```python
from build123d import *

# Parameters (mm, degrees)
BOSS_EXTRUDE1_DEPTH = 3
BOSS_EXTRUDE2_DEPTH = 10
SKETCH3_W           = 60
SKETCH3_H           = 43
CUT_EXTRUDE1_DEPTH  = 5
SKETCH4_R           = 2.5
BOSS_EXTRUDE3_DEPTH = 3.5
SKETCH5_R           = 1.3
CUT_EXTRUDE2_DEPTH  = 4.5
SKETCH6_R           = 1.3
CUT_EXTRUDE3_DEPTH  = 4.5
SKETCH7_R           = 1.3
CUT_EXTRUDE4_DEPTH  = 4.5
SKETCH8_R           = 1.3
CUT_EXTRUDE5_DEPTH  = 4.5
SKETCH9_R           = 3.1
CUT_EXTRUDE6_DEPTH  = 4.5
SKETCH10_R          = 2.5
SKETCH10_R_2        = 1.15
BOSS_EXTRUDE4_DEPTH = 8
SKETCH12_W          = 7
SKETCH12_H          = 7
BOSS_EXTRUDE5_DEPTH = 10
FILLET1_R           = 3
SKETCH13_R          = 1.3
CUT_EXTRUDE7_DEPTH  = 9


with BuildPart() as part:
    # Sketch1 → Boss-Extrude1 (new body)
    with BuildSketch(Plane(origin=(0, 0, 0), x_dir=(1, 0, 0), z_dir=(0, 1, 0))):
        with BuildLine():
            Line((70, 10), (70, -10))
            ThreePointArc((70, -10), (64.142135624, -24.142135624), (50, -30))
            Line((50, -30), (-50, -30))
            ThreePointArc((-50, -30), (-64.142135624, -24.142135624), (-70, -10))
            Line((-70, -10), (-70, 10))
            ThreePointArc((-70, 10), (-64.142135624, 24.142135624), (-50, 30))
            Line((-50, 30), (50, 30))
            ThreePointArc((50, 30), (64.142135624, 24.142135624), (70, 10))
        make_face()
    extrude(amount=BOSS_EXTRUDE1_DEPTH)

    # Sketch2 → Boss-Extrude2 (add)
    with BuildSketch(Plane(origin=(0, 3, 0), x_dir=(1, 0, 0), z_dir=(0, 1, 0))):
        with BuildLine():
            Line((-50, 30), (50, 30))
            ThreePointArc((50, 30), (64.142135624, 24.142135624), (70, 10))
            Line((70, 10), (70, -10))
            ThreePointArc((70, -10), (64.142135624, -24.142135624), (50, -30))
            Line((50, -30), (-50, -30))
            ThreePointArc((-50, -30), (-64.142135624, -24.142135624), (-70, -10))
            Line((-70, -10), (-70, 10))
            ThreePointArc((-70, 10), (-64.142135624, 24.142135624), (-50, 30))
        make_face()
        with BuildLine():
            Line((-47, 27), (47, 27))
            ThreePointArc((47, 27), (60.435028843, 21.435028843), (66, 8))
            Line((66, 8), (66, -12))
            ThreePointArc((66, -12), (59.103718437, -22.798043353), (47, -27))
            Line((47, -27), (-47, -27))
            ThreePointArc((-47, -27), (-59.103718437, -22.798043353), (-66, -12))
            Line((-66, -12), (-66, 8))
            ThreePointArc((-66, 8), (-60.435028843, 21.435028843), (-47, 27))
        make_face(mode=Mode.SUBTRACT)
    extrude(amount=BOSS_EXTRUDE2_DEPTH)

    # Sketch3 → Cut-Extrude1 (cut)
    with BuildSketch(Plane(origin=(0, 3, 0), x_dir=(1, 0, 0), z_dir=(0, 1, 0))):
        Rectangle(SKETCH3_W, SKETCH3_H)
    extrude(amount=-CUT_EXTRUDE1_DEPTH, mode=Mode.SUBTRACT)

    # Sketch4 → Boss-Extrude3 (add)
    with BuildSketch(Plane(origin=(0, 3, 0), x_dir=(1, 0, 0), z_dir=(0, 1, 0))):
        with Locations((-33.75, 18.25)):
            Circle(SKETCH4_R)
        with Locations((-33.75, -18.25)):
            Circle(SKETCH4_R)
        with Locations((32.75, -18.25)):
            Circle(SKETCH4_R)
        with Locations((32.75, 18.25)):
            Circle(SKETCH4_R)
    extrude(amount=BOSS_EXTRUDE3_DEPTH)

    # Sketch5 → Cut-Extrude2 (cut)
    with BuildSketch(Plane(origin=(0, 6.5, 0), x_dir=(1, 0, 0), z_dir=(0, 1, 0))):
        with Locations((-33.75, -18.25)):
            Circle(SKETCH5_R)
    extrude(amount=-CUT_EXTRUDE2_DEPTH, mode=Mode.SUBTRACT)

    # Sketch6 → Cut-Extrude3 (cut)
    with BuildSketch(Plane(origin=(0, 6.5, 0), x_dir=(1, 0, 0), z_dir=(0, 1, 0))):
        with Locations((-33.75, 18.25)):
            Circle(SKETCH6_R)
    extrude(amount=-CUT_EXTRUDE3_DEPTH, mode=Mode.SUBTRACT)

    # Sketch7 → Cut-Extrude4 (cut)
    with BuildSketch(Plane(origin=(0, 6.5, 0), x_dir=(1, 0, 0), z_dir=(0, 1, 0))):
        with Locations((32.75, 18.25)):
            Circle(SKETCH7_R)
    extrude(amount=-CUT_EXTRUDE4_DEPTH, mode=Mode.SUBTRACT)

    # Sketch8 → Cut-Extrude5 (cut)
    with BuildSketch(Plane(origin=(0, 6.5, 0), x_dir=(1, 0, 0), z_dir=(0, 1, 0))):
        with Locations((32.75, -18.25)):
            Circle(SKETCH8_R)
    extrude(amount=-CUT_EXTRUDE5_DEPTH, mode=Mode.SUBTRACT)

    # Sketch9 → Cut-Extrude6 (cut)
    with BuildSketch(Plane(origin=(0, 3, 0), x_dir=(1, 0, 0), z_dir=(0, 1, 0))):
        with Locations((-44, 0.1)):
            Circle(SKETCH9_R)
        with Locations((-52.1, 8.2)):
            Circle(SKETCH9_R)
        with Locations((-60.2, 0.1)):
            Circle(SKETCH9_R)
        with Locations((-52.1, -8)):
            Circle(SKETCH9_R)
        Polygon((62.3, 3.2), (54.2, 3.2), (54.2, 5.1), (54.2, 11.3), (48, 11.3), (48, 5.1), (48, 3.2), (46.1, 3.2), (39.9, 3.2), (39.9, -3), (46.1, -3), (48, -3), (48, -4.9), (48, -11.1), (54.2, -11.1), (54.2, -4.9), (54.2, -3), (62.3, -3), align=None)
    extrude(amount=-CUT_EXTRUDE6_DEPTH, mode=Mode.SUBTRACT)

    # Sketch10 → Boss-Extrude4 (add)
    with BuildSketch(Plane(origin=(0, 3, 0), x_dir=(1, 0, 0), z_dir=(0, 1, 0))):
        with Locations((-52.1, -16.1)):
            Circle(SKETCH10_R)
        with Locations((-52.1, -16.1)):
            Circle(SKETCH10_R_2, mode=Mode.SUBTRACT)
        with Locations((-52.1, 16.3)):
            Circle(SKETCH10_R)
        with Locations((-52.1, 16.3)):
            Circle(SKETCH10_R_2, mode=Mode.SUBTRACT)
        with Locations((51.1, 16.3)):
            Circle(SKETCH10_R)
        with Locations((51.1, 16.3)):
            Circle(SKETCH10_R_2, mode=Mode.SUBTRACT)
        with Locations((51.1, -16.1)):
            Circle(SKETCH10_R)
        with Locations((51.1, -16.1)):
            Circle(SKETCH10_R_2, mode=Mode.SUBTRACT)
    extrude(amount=BOSS_EXTRUDE4_DEPTH)

    # Sketch12 → Boss-Extrude5 (add)
    with BuildSketch(Plane(origin=(0, 3, 0), x_dir=(1, 0, 0), z_dir=(0, 1, 0))):
        with Locations((-43.5, 23.5)):
            Rectangle(SKETCH12_W, SKETCH12_H)
        with Locations((-43.5, -23.5)):
            Rectangle(SKETCH12_W, SKETCH12_H)
        with Locations((43.5, -23.5)):
            Rectangle(SKETCH12_W, SKETCH12_H)
        with Locations((43.5, 23.5)):
            Rectangle(SKETCH12_W, SKETCH12_H)
    extrude(amount=BOSS_EXTRUDE5_DEPTH)

    # Fillet1
    fillet1_edges = [part.edges().sort_by_distance(p)[0] for p in [
        (70, 0, 0),
        (64.142135624, 0, 24.142135624),
        (0, 0, 30),
        (-64.142135624, 0, 24.142135624),
        (-70, 0, 0),
        (-64.142135624, 0, -24.142135624),
        (0, 0, -30),
        (64.142135624, 0, -24.142135624),
    ]]
    fillet(fillet1_edges, radius=FILLET1_R)

    # Sketch13 → Cut-Extrude7 (cut)
    with BuildSketch(Plane(origin=(0, 13, 0), x_dir=(1, 0, 0), z_dir=(0, 1, 0))):
        with Locations((-43.5, 23.5)):
            Circle(SKETCH13_R)
        with Locations((-43.5, -23.5)):
            Circle(SKETCH13_R)
        with Locations((43.5, -23.5)):
            Circle(SKETCH13_R)
        with Locations((43.5, 23.5)):
            Circle(SKETCH13_R)
    extrude(amount=-CUT_EXTRUDE7_DEPTH, mode=Mode.SUBTRACT)


solid = part.part
```
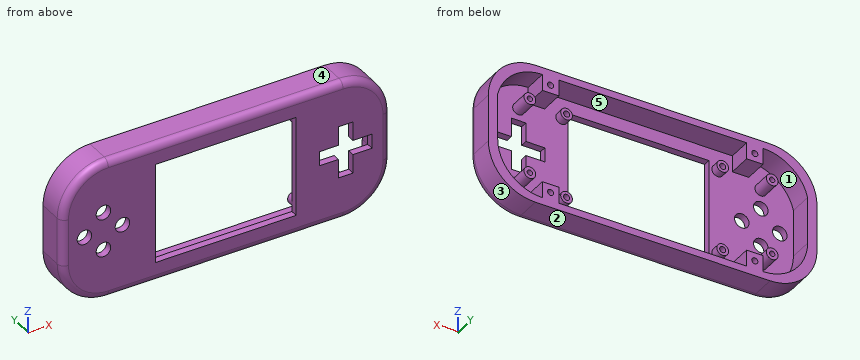
Part model, mm, in its own coordinate system. Face numbers are marked on the shaded views. A direction names the side the tool comes from. Coordinates: 2 decimals unless noted, no trailing zeros. Loops run counter-clockwise (first coordinate to the right, second up) from the corner with the lowest first, then second, coordinate; pieces in that order, holes last. Notation, with made-up numbers: (-35.5, -22.5) - (-29.5, -22.5) arc R21 ccw to (-29.5, -2.5) - close; hole circle Ø5 at (-20.75, -24.5). An arc over 180 degrees is marked (long way). Write item = value, one per line. Start each with the question number.
Item 1: Wall check: L1, parallel to Z at x = -33.75, y = 5.05; L2, parallel to Z at x = 43.5, y = 7.5; L3, parallel to X at y = 10.5, z = 4.5. Give the ranges that are in metal, low to high. Write a range as from..to.
Item 2: Cut at D-D, the plane x = -43.5. Give the cut face in (y, z).
Item 3: Mould opens along X. For the marked faces 1, 2 and 3 say: released by +X, released by -X, zero draft, split by the parting line, or undercut.
Item 4: Cut at B-B, the plane z = 8. Give the cut face in (x, y).
Item 5: Cut at C-C, the plane x = 32.75. Give the cut face in (y, z), and give its area (3 significant figures).
Item 6: Cut at A-A, the plane x = -9.5. Give the cut face in (y, z), and give its area (3 significant figures).
Item 7: Flat gauge pins, fed straight in: pin 1 Ø2 at (y, z) = (8, 23) entering from -X; pin 2 Ø1 at (x, z) = (-47, 0) entering from -Y; pin 3 Ø1.5 at (x, z) = (50.5, -15.5) entering from +Y; pin 4 Ø0.9 at (y, z) = (1, -7.5) entering from +X. Where does each tip first touch, or does it go through?
Item 8: 3-axis set-ups, long thin cutter, end or side, ignore diameter. For the marked faces 4 and 5: which of +Z, -Z, +X, -X, +Y, -Y reach the whole face in a straight line?
The answers:
q1.L1 = -30..-27, -20.75..-19.55, -16.95..-15.75, 15.75..16.95, 19.55..20.75, 27..30
q1.L2 = -30..-24.8, -22.2..-20, 20..22.2, 24.8..30
q1.L3 = -70..-66, 66..70
q2.outline = (0, -27) arc R3 ccw to (3, -30) - (13, -30) - (13, -24.8) - (4, -24.8) - (4, -22.2) - (13, -22.2) - (13, -20) - (3, -20) - (3, -3.16) - (0, -3.16) - close; (0, 2.96) - (3, 2.96) - (3, 20) - (13, 20) - (13, 22.2) - (4, 22.2) - (4, 24.8) - (13, 24.8) - (13, 30) - (3, 30) arc R3 ccw to (0, 27) - close
q3.face_1 = undercut
q3.face_2 = zero draft
q3.face_3 = released by +X
q4.outline = (-70, 3) arc R3 ccw to (-67, 0) - (-55.2, 0) - (-55.2, 3) - (-66, 3) - (-66, 13) - (-70, 13) - close; (-49, 0) - (-30, 0) - (-30, 3) - (-49, 3) - close; (30, 0) - (48, 0) - (48, 3) - (30, 3) - close; (54.2, 0) - (67, 0) arc R3 ccw to (70, 3) - (70, 13) - (66, 13) - (66, 3) - (54.2, 3) - close
q5.outline = (0, -27) arc R3 ccw to (3, -30) - (13, -30) - (13, -27) - (3, -27) - (3, -20.75) - (6.5, -20.75) - (6.5, -19.55) - (2, -19.55) - (2, -16.95) - (6.5, -16.95) - (6.5, -15.75) - (3, -15.75) - (3, 15.75) - (6.5, 15.75) - (6.5, 16.95) - (2, 16.95) - (2, 19.55) - (6.5, 19.55) - (6.5, 20.75) - (3, 20.75) - (3, 27) - (13, 27) - (13, 30) - (3, 30) arc R3 ccw to (0, 27) - close
q5.area = 248 mm2
q6.outline = (0, -27) arc R3 ccw to (3, -30) - (13, -30) - (13, -27) - (3, -27) - (3, -21.5) - (0, -21.5) - close; (0, 21.5) - (3, 21.5) - (3, 27) - (13, 27) - (13, 30) - (3, 30) arc R3 ccw to (0, 27) - close
q6.area = 107 mm2
q7.pin_1 = -66
q7.pin_2 = 0
q7.pin_3 = 11
q7.pin_4 = 69.57
q8.face_4 = +Z, +X, -X, +Y, -Y
q8.face_5 = +Y
